from build123d import *

# Parameters (mm, degrees)
F1_DEPTH = 88.9
F2_R     = 2.2479
F3_DEPTH = 5.842
F4_START = -82.55
F4_DEPTH = 6.35


with BuildPart() as f1:
    # F0 (on Front) → F1 (new body)
    with BuildSketch(Plane.XZ):
        with BuildLine():
            Line((26.9766840256, 11.7828417273), (30.0785363078, 11.7828417273))
            ThreePointArc((30.0785363078, 11.7828417273), (-36.5136837388, 75.1364181979), (-103.1059037855, 11.7828417273))
            Line((-103.1059037855, 11.7828417273), (-100.0040515032, 11.7828417273))
            Line((-100.0040515032, 11.7828417273), (-96.7471775005, 11.7828417273))
            ThreePointArc((-96.7471775005, 11.7828417273), (-36.5136837388, 68.7864181979), (23.7198100229, 11.7828417273))
            Line((23.7198100229, 11.7828417273), (26.9766840256, 11.7828417273))
        make_face()
        with BuildLine():
            Line((-100.0040515032, 11.7828417273), (-103.1059037855, 11.7828417273))
            ThreePointArc((-103.1059037855, 11.7828417273), (-103.1634009398, 10.2973980525), (-103.1877670725, 8.8110417273))
            Line((-103.1877670725, 8.8110417273), (-100.0040515032, 8.8110417273))
            Line((-100.0040515032, 8.8110417273), (-100.0040515032, 11.7828417273))
        make_face()
        with BuildLine():
            Line((26.9766840256, 8.8110417273), (30.1603995949, 8.8110417273))
            ThreePointArc((30.1603995949, 8.8110417273), (30.1360334622, 10.2973980525), (30.0785363078, 11.7828417273))
            Line((30.0785363078, 11.7828417273), (26.9766840256, 11.7828417273))
            Line((26.9766840256, 11.7828417273), (26.9766840256, 8.8110417273))
        make_face()
        with BuildLine():
            Line((30.1603995949, 8.8110417273), (33.335441262, 8.8110417273))
            ThreePointArc((33.335441262, 8.8110417273), (33.312184154, 10.2973574694), (33.2573033958, 11.7828417273))
            Line((33.2573033958, 11.7828417273), (30.0785363078, 11.7828417273))
            ThreePointArc((30.0785363078, 11.7828417273), (30.1360334622, 10.2973980525), (30.1603995949, 8.8110417273))
        make_face()
        with BuildLine():
            Line((30.0785363078, 11.7828417273), (33.2573033958, 11.7828417273))
            ThreePointArc((33.2573033958, 11.7828417273), (-36.5136837388, 78.3114181979), (-106.2846708734, 11.7828417273))
            Line((-106.2846708734, 11.7828417273), (-103.1059037855, 11.7828417273))
            ThreePointArc((-103.1059037855, 11.7828417273), (-36.5136837388, 75.1364181979), (30.0785363078, 11.7828417273))
        make_face()
        with BuildLine():
            Line((-103.1059037855, 11.7828417273), (-106.2846708734, 11.7828417273))
            ThreePointArc((-106.2846708734, 11.7828417273), (-106.3395516317, 10.2973574694), (-106.3628087397, 8.8110417273))
            Line((-106.3628087397, 8.8110417273), (-103.1877670725, 8.8110417273))
            ThreePointArc((-103.1877670725, 8.8110417273), (-103.1634009398, 10.2973980525), (-103.1059037855, 11.7828417273))
        make_face()
    extrude(amount=F1_DEPTH)

    # F2 (on face) → F3 (join)
    with BuildSketch(Plane.XZ.offset(88.9)):
        with Locations((-36.5136837388, 73.5362181979)):
            Circle(F2_R)
        with Locations((9.5011486255, 54.4762505622)):
            Circle(F2_R)
        with Locations((-82.5285161032, 54.4762505622)):
            Circle(F2_R)
    extrude(amount=F3_DEPTH)

    # F2 (on face) → F4 (cut)
    with BuildSketch(Plane.XZ.offset(88.9).offset(F4_START)):
        with Locations((-82.5285161032, 54.4762505622)):
            Circle(F2_R)
        with Locations((-36.5136837388, 73.5362181979)):
            Circle(F2_R)
        with Locations((9.5011486255, 54.4762505622)):
            Circle(F2_R)
    extrude(amount=-F4_DEPTH, mode=Mode.SUBTRACT)


solid = f1.part
Can you work these out from the model? Positions are in its coordinate system, mm. A direction names the side the tool comes from. Give positions to 0.01 mm unless a question says otherwise; leave off trailing zeros. Order: outer loops, then holes, each group sorted by start corner. A loop starts at its lowest first (then second) coordinate and runs counter-clockwise, first axis right, second up. Notation, with made-up numbers: M 6.5,-33.75 L 45.5,-33.75 A27 ccw 45.5,-13.75 Z; hole C -4.75,-32.5 d8. An arc over 180 degrees is marked long. Use a Markdown table: item, result. Add a question column.
Item 1: Suppose I cut it at D-D (x = -31.5). List the corners of the cut face in (y, z) for me.
Item 2: For faces 5 (the flat face through (-37, -6.35, 74)), 6 (the cylindrical face through (-80.4, -91.8, 55.2)), 7 (the flat face through (-98, -44, 11.783)), which set-ups out of +Z, -Z, +X, -X, +Y, -Y let a thin tool reach every point of the face, with its end or its side?
Item 3: We'd pull the mould along Z, two halves only. Please class faces 1 (the cylindrical face through (-35.48, -3.22, 71.54)), 2 (the flat face through (30, -44, 8.811)), 3 (the cylindrical face through (-80.4, -3.2, 55.2)), 4 (the cylindrical face through (9.014, -91.78, 52.282)): +Z half, -Z half, draft (parallel to the pull), parting line (faces both ways), or undercut.
Item 4: Suppose I cut it at B-B (y = -47). List the corners of the cut face in (x, z) for me (3 decimals), then the cut area to 3 significant figures.
Item 5: Suppose I cut it at A-A (z = 27). List the corners of the cut face in (x, y) for me, then the cut area to 3 significant figures.
Item 6: Suppose I cut it at C-C (z = 47). List the corners of the cut face in (x, y) for me.
Item 7: Will these pins go through, and if not, where does the flat tip stop? pin 1 (1.3 mm diameter, centred on x = -36, z = 72.5, fed in from +Y); pin 2 (1 mm diameter, centred on x = -97.5, y = -41, fed in from -Z); pin 3 (12 mm diameter, centred on x = -57.5, y = -30, fed in from +Z).
Item 8: If I drill on L1, parallel to X at y = -13.5, z = 38.5; L2, parallel to X at y = -76, z = 44.5; L3, parallel to Y at x = 24.5, z = 34, over which ranges is the centre line in solid material (lowest first)? Write a range as [from, to].
Answer sheet:
| question | item | result |
|---|---|---|
| 1 | outline | M -88.9,68.58 L 0,68.58 L 0,78.13 L -88.9,78.13 Z |
| 2 | face 5 | +Y |
| 2 | face 6 | -Y |
| 2 | face 7 | -Z, +Y, -Y |
| 3 | face 1 | undercut |
| 3 | face 2 | -Z half |
| 3 | face 3 | undercut |
| 3 | face 4 | parting line |
| 4 | outline | M -106.363,8.811 L -100.004,8.811 L -100.004,11.783 L -96.747,11.783 A60.325 cw 23.72,11.783 L 26.977,11.783 L 26.977,8.811 L 33.335,8.811 A69.85 ccw Z |
| 4 | area | 1,920 mm² |
| 5 | outline | M -103.86,-88.9 L -93.92,-88.9 L -93.92,0 L -103.86,0 Z; M 20.89,-88.9 L 30.83,-88.9 L 30.83,0 L 20.89,0 Z |
| 5 | area | 1,770 mm² |
| 6 | outline | M -94.77,-88.9 L -82.92,-88.9 L -82.92,0 L -94.77,0 Z; M 9.9,-88.9 L 21.74,-88.9 L 21.74,0 L 9.9,0 Z |
| 7 | pin 1 | stops at y = -6.35 |
| 7 | pin 2 | stops at z = 11.78 |
| 7 | pin 3 | stops at z = 76.68 |
| 8 | L1 | x = [-99.57, -88.83], [15.8, 26.55] |
| 8 | L2 | x = [-96.35, -84.89], [11.86, 23.32] |
| 8 | L3 | y = [-88.9, 0] |
